from build123d import *

# Parameters (mm, degrees)
F1_DEPTH = 11
F2_R     = 8
F3_W     = 12.6
F3_H     = 5.3
F4_DEPTH = 25
F5_W     = 7.9238843173
F5_H     = 2.3
F6_DEPTH = 25


with BuildPart() as f1:
    # F0 (on Top) → F1 (new body, symmetric)
    with BuildSketch(Plane.XY):
        with BuildLine():
            Line((-38.625, -21.65), (38.625, -21.65))
            ThreePointArc((38.625, -21.65), (44.2818542495, -19.3068542495), (46.625, -13.65))
            Line((46.625, -13.65), (46.625, 13.65))
            ThreePointArc((46.625, 13.65), (44.2818542495, 19.3068542495), (38.625, 21.65))
            Line((38.625, 21.65), (-38.625, 21.65))
            ThreePointArc((-38.625, 21.65), (-44.2818542495, 19.3068542495), (-46.625, 13.65))
            Line((-46.625, 13.65), (-46.625, -13.65))
            ThreePointArc((-46.625, -13.65), (-44.2818542495, -19.3068542495), (-38.625, -21.65))
        make_face()
    extrude(amount=F1_DEPTH, both=True)

    # F2
    f2_edges = [f1.edges().sort_by_distance(p)[0] for p in [
        (0, -21.65, 11),
        (44.281854, -19.306854, 11),
        (46.625, 0, 11),
        (44.281854, 19.306854, 11),
        (0, 21.65, 11),
        (-44.281854, 19.306854, 11),
        (-46.625, 0, 11),
        (-44.281854, -19.306854, 11),
        (0, -21.65, -11),
        (44.281854, -19.306854, -11),
        (46.625, 0, -11),
        (44.281854, 19.306854, -11),
        (0, 21.65, -11),
        (-44.281854, 19.306854, -11),
        (-46.625, 0, -11),
        (-44.281854, -19.306854, -11),
    ]]
    fillet(f2_edges, radius=F2_R)

    # F3 (on face) → F4 (cut)
    with BuildSketch(Plane(origin=(-46.625, 0, 0), x_dir=(0, -1, 0), z_dir=(-1, 0, 0))):
        with Locations((-5.15, 1.15)):
            Rectangle(F3_W, F3_H)
    extrude(amount=-F4_DEPTH, mode=Mode.SUBTRACT)

    # F5 (on face) → F6 (cut)
    with BuildSketch(Plane(origin=(0, 21.65, 0), x_dir=(-1, 0, 0), z_dir=(0, 1, 0))):
        with Locations((32.0630578414, -0.65)):
            Rectangle(F5_W, F5_H)
    extrude(amount=-F6_DEPTH, mode=Mode.SUBTRACT)


solid = f1.part
For this review, take the finished solid that the model builds, in its own axes (mm). A direction names the side the tool comes from. Round coordinates to 2 decimals unless told otherwise and drop trailing zeros. Order: outer loops, then holes, each group sorted by start corner. A loop starts at its lowest first (then second) coordinate and runs counter-clockwise, first axis right, second up. Notation, with made-up numbers: M 28,86.25 L 47,86.25 A32 ccw 47,116.25 Z; hole C 61,6.25 d3. An arc over 180 degrees is marked long. Use a Markdown table: item, result. Add a question column.
Item 1: Insertion check: pin 1 (14 mm diameter, centred on x = -39, y = 4.5, fed in from -Z); pin 2 (1 mm diameter, centred on x = -19.5, z = 4, fed in from -Y); pin 3 (3 mm diameter, centred on y = 6, z = 3, fed in from -X); pin 4 (0.7 mm diameter, centred on y = 5.5, z = 0, fed in from -X) (3 decimals). Each pin has a flat end and moves straight along its axis. Give the tip position at first contact, or say it passes through.
Item 2: Add section D-D, the plane z = -4.5. Give the boundary of the cut face in (x, y) (3 decimals).
Item 3: Add section B-B, the plane x = -9. Give the boundary of the cut face in (y, z), then the cut area to 3 significant figures.
Item 4: To check wall thickness, follow line 1 along Z through (x, y) = (-37, 0); line 2 along X through (y, z) = (11.5, -0.5) (3 decimals); line 3 along X through (y, z) = (4, 2.25) (3 decimals). State the ranges of each line that lie inside material, in increasing order.
Item 5: Add section A-A, the plane x = -22.5. Give the boundary of the cut face in (y, z).
Item 6: Add section C-C, the plane y = 10.5. Give the boundary of the cut face in (x, z) (3 decimals).
Item 7: Mouldability with a two-part tool opening along Y and no side actions: class faces 1 (the cylindrical face through (-0.541, 19.369, -8.594)), 2 (the flat face through (-34, 5, 3.8)), 3 (the flat face through (-1, 0, -11)) as released by +Y, released by -Y, zero draft, split by the parting line, or undercut.
Item 8: Tool access review of faces 4 (the flat face through (-41, 5, -1.5)), 5 (the cylindrical face through (-44.344, -0.191, 8.594)), 6 (the flat face through (-36.025, 12, -1)): name each direction out of +Z, -Z, +X, -X, +Y, -Y from which nothing blocks a thin tool from reaching the whole face with its end or side.
Geometry results:
| question | item | result |
|---|---|---|
| 1 | pin 1 | stops at z = -11 |
| 1 | pin 2 | stops at y = -21.63 |
| 1 | pin 3 | stops at x = -46.58 |
| 1 | pin 4 | stops at x = -21.625 |
| 2 | outline | M -46.483,-13.65 A7.858 ccw -38.625,-21.508 L 38.625,-21.508 A7.858 ccw 46.483,-13.65 L 46.483,13.65 A7.858 ccw 38.625,21.508 L -38.625,21.508 A7.858 ccw -46.483,13.65 Z |
| 3 | outline | M -21.65,-3 A8 ccw -13.65,-11 L 13.65,-11 A8 ccw 21.65,-3 L 21.65,3 A8 ccw 13.65,11 L -13.65,11 A8 ccw -21.65,3 Z |
| 3 | area | 898 mm² |
| 4 | line 1 | z = -11 to -1.5, 3.8 to 11 |
| 4 | line 2 | x = -46.625 to -36.025, -28.101 to 46.625 |
| 4 | line 3 | x = -21.625 to 46.625 |
| 5 | outline | M -21.65,-3 A8 ccw -13.65,-11 L 13.65,-11 A8 ccw 21.65,-3 L 21.65,3 A8 ccw 13.65,11 L -13.65,11 A8 ccw -21.65,3 Z; hole M -1.15,-1.5 L 11.45,-1.5 L 11.45,3.8 L -1.15,3.8 Z |
| 6 | outline | M -46.625,-3 A8 ccw -38.625,-11 L 38.625,-11 A8 ccw 46.625,-3 L 46.625,3 A8 ccw 38.625,11 L -38.625,11 A8 ccw -46.585,3.8 L -21.625,3.8 L -21.625,-1.5 L -28.101,-1.5 L -28.101,-1.8 L -36.025,-1.8 L -36.025,-1.5 L -46.625,-1.5 Z |
| 7 | face 1 | released by +Y |
| 7 | face 2 | undercut |
| 7 | face 3 | zero draft |
| 8 | face 4 | -X |
| 8 | face 5 | +Z, -X, +Y, -Y |
| 8 | face 6 | +Y |
